Could you check a few things on this model? Use its own coordinates, in mm. A direction names the side the tool comes from. Round coordinates to 2 decimals unless told otherwise and drop trailing zeros. Loops run counter-clockwise (first coordinate to the right, second up) from the corner with the lowest first, then second, coordinate; pieces in that order, holes last. Notation, with made-up numbers: (50.25, 24) -> (106.25, 24) arc R29 cw to (106.25, 50) -> close; hole circle Ø1 at (69, 49). An arc over 180 degrees is marked (long way). Write each question's results on one line, items separated by ' | '. Start each with the question number.
1) Imagine slicing it at A-A, the plane z = -88. List the corners of the cut face in (x, y) for me, plus the area to 3 significant figures.
2) Imagine slicing it at C-C, the plane x = -29.45. List the corners of the cut face in (y, z) for me, plus the area to 3 significant figures.
3) Imagine slicing it at D-D, the plane y = 22.5. List the corners of the cut face in (x, z) for me, plus the area to 3 significant figures.
4) If I drill on probe 1 along X at (y, z) = (1, -4); probe 2 along Z at (x, y) = (-106, 1.75); probe 3 along Z at (x, y) = (-106, 0.45), over which ranges is the centre line in solid material (lowest first)?
5) Imagine slicing it at B-B, the plane y = 5. List the corners of the cut face in (x, z) for me, plus the area to 3 significant figures.
6) Which directions (+Z, -Z, +X, -X, +Y, -Y) give clear straight access to the entire face, cutting with the end or side of a thin tool? Please do faces 1 (the flat face through (-33.9, 5, -79)), 2 (the flat face through (-25, 5, -79)), 3 (the flat face through (-29, 5, -75.5)).
7) We'd pull the mould along Z, two halves only. Please class faces 4 (the flat face through (-30, 5, -82.5)), 5 (the cylindrical face through (-28.164, 4.451, -78.331)), 6 (the cylindrical face through (-0.9, 1.01, -0.86)), 7 (the flat face through (-30, 8, -77)): pulls with the +Z half, pulls with the -Z half, needs draft (parallel to the pull), parting line crosses it, or undercut.
8) For P1, Ø6, axis at x = -106, z = -4, coming from the +Y side; P2, Ø3, axis at x = -49, y = 20.5, coming from the +Z side; P3, Ø1.5, axis at x = -54, y = 16.5, coming from the -Z side, each with a flat end and sliding along its axis, tell me the tip position at first contact or that it passes through.
Autodesk Inventor part; units mm, degrees
ref_plane "Płaszczyzna konstrukcyjna2" through (-100, 0, -97) normal (-1, 0, 0) x (0, 0, 1)
ref_plane "YZ Plane" through (0, 0, 0) normal (1, 0, 0) x (0, 1, 0)
ref_plane "XZ Plane" through (0, 0, 0) normal (0, 1, 0) x (-1, 0, 0)
sketch "Szkic1" plane through (0, 0, 0) normal (0, 1, 0) x (-1, 0, 0)
  line L0 (110, 0) -> (0, 0)
  line L1 (0, 0) -> (0, -100)
  line L2 (0, -100) -> (110, -100)
  line L3 (110, -100) -> (110, 0)
  dimension "d0" = 100
  dimension "d1" = 110
extrude "Gabaryt" add sketch "Szkic1" along normal blind 2
sketch "Szkic2" plane through (0, 0, 0) normal (0, 1, 0) x (1, 0, 0)
  line L0 (0, 0) -> (0, 100)
  line L1 (-110, 0) -> (0, 0)
  line L2 (-110, 100) -> (-110, 0)
  line L3 (0, 100) -> (-110, 100)
  line L4 (-110, 50) -> (0, 50)
  line L5 (-55, 100) -> (-55, 0)
  point P0 (-4, 4)
  point P1 (-106, 4)
  point P2 (-4, 96)
  point P3 (-106, 96)
  dimension "d4" = 4
  dimension "d5" = 4
hole "Otwory montażowe" at (-4, 0, -4) at (-106, 0, -4) at (-106, 0, -96) at (-4, 0, -96) direction (0, 1, 0) diameter 2.6 end through all counterbore diameter 4.5 counterbore depth 1.5
fillet "Zaokrąglenie1" radius 3 4 edges at (0, 1, 0) (-110, 1, 0) (-110, 1, -100) (0, 1, -100)
ref_plane "Płaszczyzna konstrukcyjna2" through (-100, 0, -97) normal (-1, 0, 0) x (0, 0, 1)
sketch "Szkic4" plane through (-100, 0, -97) normal (-1, 0, 0) x (0, 0, 1)
  line L0 (0, 2) -> (94, 2)
  line L1 (0, 28.3) -> (2, 28.3)
  line L2 (2, 28.3) -> (2, 2)
  line L3 (2, 2) -> (0, 2)
  line L4 (0, 2) -> (0, 28.3)
  line L5 (19.5, 28.3) -> (21.5, 28.3)
  line L6 (21.5, 28.3) -> (21.5, 2)
  line L7 (21.5, 2) -> (19.5, 2)
  line L8 (19.5, 2) -> (19.5, 28.3)
  line L9 (0, 30.3) -> (21.5, 30.3)
  line L10 (21.5, 30.3) -> (21.5, 28.3)
  line L11 (21.5, 28.3) -> (0, 28.3)
  line L12 (0, 28.3) -> (0, 30.3)
  line L13 (-3, 2) -> (-3, 0)
  point P0 (97, 0)
  point P1 (2, 2)
  point P2 (2, 28.3)
  point P3 (19.5, 2)
  point P4 (21.5, 2)
  dimension "d20" = 2
  dimension "d21" = 2
  dimension "d22" = 2
  dimension "d23" = 17.5
  dimension "d24" = 26.3
  dimension "d25" = 3
extrude "Wyciągnięcie proste3" add sketch "Szkic4" against normal blind 55 contours L4 L1 L2 L0 | L12 L9 L10 L5 L11 L1 | L8 L5 L6 L0
sketch "Szkic5" plane through (0, 2, 0) normal (0, 1, 0) x (1, 0, 0)
  line L0 (-33.9, 82.5) -> (-25, 82.5)
  line L1 (-25, 82.5) -> (-25, 75.5)
  line L2 (-25, 75.5) -> (-33.9, 75.5)
  line L3 (-33.9, 75.5) -> (-33.9, 82.5)
  line L4 (-100, 75.5) -> (-45, 75.5)
  line L5 (-110, 97) -> (-110, 3)
  line L6 (0, 3) -> (0, 97)
  point P0 (0, 0)
  point P1 (-29.45, 82.5)
  dimension "d28" = 7
  dimension "d29" = 8.9
  dimension "d34" = 25
extrude "Wyciągnięcie proste4" add sketch "Szkic5" along normal blind 6
sketch "Szkic6" plane through (0, 8, 0) normal (0, 1, 0) x (1, 0, 0)
  line L0 (-25, 82.5) -> (-33.9, 82.5)
  line L1 (-33.9, 82.5) -> (-33.9, 75.5)
  line L2 (-33.9, 75.5) -> (-25, 75.5)
  line L3 (-25, 75.5) -> (-25, 82.5)
  line L4 (-33.9, 75.5) -> (-33.9, 82.5)
  line L5 (-33.9, 79) -> (-25, 79)
  line L6 (-29.45, 82.5) -> (-29.45, 75.5)
  point P0 (0, 0)
  point P1 (-29.45, 79)
hole "Otwór2" at (-29.45, 8, -79) direction (0, -1, 0) diameter 2.9 depth 7
equation "\"d0\" = podstawa_a"
equation "\"d1\" = podstawa_b"
equation "\"d2\" = podstawa_wys"
equation "\"d6\" = gniazdo_M2_D2"
equation "\"d8\" = gniazdo_M2_D1"
equation "\"d9\" = gniazdo_M2_glebokosc"
equation "\"d13\" = podstawa_zaokraglenie"
equation "\"d20\" = obudowa_uchwyt_grubosc"
equation "\"d21\" = d20"
equation "\"d22\" = d20"
equation "\"d23\" = obudowa_uchwyt_szerokosc_wew"
equation "\"d24\" = obudowa_uchwyt_wysokosc_wew"
equation "\"d25\" = obudowa_uchwyt_poz_z"
equation "\"d26\" = obudowa_uchwyt_kolnierz_wys"
equation "\"d28\" = podstawa_mocowanie_DC_a"
equation "\"d29\" = podstawa_mocowanie_DC_b"
equation "\"d34\" = obudowa_gniazdo_poz"
equation "\"d32\" = podstawa_mocowanie_DC_wys"
equation "\"d35\" = insert_D"
equation "\"d37\" = gniazdo_M2_D1"
equation "\"d38\" = gniazdo_M2_glebokosc"
equation "\"d40\" = insert_glebokosc"
equation "\"podstawa_a\" = 100"
equation "\"podstawa_b\" = 110"
equation "\"podstawa_wys\" = 2"
equation "\"podstawa_otwory_montazowe_poz_y\" = 4"
equation "\"podstawa_otwory_montazowe_poz_x\" = 4"
equation "\"gniazdo_M2_D1\" = 4.5"
equation "\"gniazdo_M2_glebokosc\" = 1.5"
equation "\"gniazdo_M2_D2\" = 2.6"
equation "\"obudowa_wys\" = 45"
equation "\"obudowa_grubosc\" = 2"
equation "\"obudowa_prowadnica_odsuniecie\" = 2"
equation "\"obudowa_prowadnica_grubosc\" = 2"
equation "\"obudowa_kontrolki_a\" = 38"
equation "\"obudowa_prowadnica_wys\" = 19"
equation "\"obudowa_otwory_montazowe_poz_y\" = 4"
equation "\"obudowa_otwory_montazowe_poz_x\" = 4"
equation "\"obudowa_otwory_montazowe_material_y\" = 8"
equation "\"obudowa_otwory_montazowe_material_x\" = 8"
equation "\"insert_D\" = 2.9"
equation "\"insert_glebokosc\" = 7"
equation "\"obudowa_zaokraglenie\" = 3"
equation "\"podstawa_zaokraglenie\" = 3"
equation "\"obudowa_otwory_io_wys\" = 15"
equation "\"obudowa_otwory_io_D\" = 15"
equation "\"obudowa_otwory_io1_poz\" = 55"
equation "\"obudowa_otwory_io1_wys\" = 25"
equation "\"obudowa_otwory_io1_D\" = 12"
equation "\"obudowa_otwory_io2_poz\" = 38"
equation "\"obudowa_otwory_io2_wys\" = 25"
equation "\"obudowa_otwory_io2_D\" = 12"
equation "\"obudowa_otwory_pot_D\" = 7.2"
equation "\"input_b\" = 14.4"
equation "\"input_wys\" = 10.9"
equation "\"input_a\" = 8.9"
equation "\"obudowa_MTS_otwor_D\" = 6.2"
equation "\"obudowa_pot_poz_y\" = 15"
equation "\"obudowa_s_poz_x\" = 78"
equation "\"obudowa_s_D\" = 6.2"
equation "\"obudowa_s_poz_y\" = 15"
equation "\"obudowa_s_rozstaw_y\" = 16"
equation "\"pcb_rozstaw_x\" = 92"
equation "\"pcb_rozstaw_y\" = 58"
equation "\"obudowa_pcb_grubosc_scianki\" = 6"
equation "\"pcb_grubosc_scianki\" = 6"
equation "\"pcb_poz_y\" = 29"
equation "\"pcb_wys_bloku\" = 35"
equation "\"obudowa_footswitch_poz_y\" = 68"
equation "\"obudowa_footswitch_poz_x\" = 35"
equation "\"obudowa_footswitch_D\" = 12.3"
equation "\"obudowa_led_indicator_D\" = 3.5"
equation "\"obudowa_led_indicator_poz_x\" = 55"
equation "\"obudowa_podkladka_otwory\" = 4"
equation "\"podstawa_uchwyt_grubosc\" = 3"
equation "\"podstawa_uchwyt_wysokosc\" = 15"
equation "\"obudowa_uchwyt_grubosc\" = 2"
equation "\"pbudowa_uchwyt_podciecie_wys\" = 1.5"
equation "\"obudowa_uchwyt_wysokosc_wew\" = 26.3"
equation "\"obudowa_uchwyt_szerokosc_wew\" = 17.5"
equation "\"obudowa_gniazdo_poz\" = 25"
equation "\"obudowa_uchwyt_kolnierz_wys\" = 55"
equation "\"obudowa_uchwyt_poz_y\" = 2"
equation "\"obudowa_uchwyt_poz_z\" = 3"
equation "\"obudowa_podciecie_inout_wys\" = 6"
equation "\"obudowa_podciecie_logo_wys\" = 34"
equation "\"obudowa_podciecie_logo_szerokosc\" = 25"
equation "\"obudowa_pot_pozycjonowanie_wys\" = 13"
equation "\"obudowa_pot_pozycjonowanie_szerokosc\" = 2.8"
equation "\"obudowa_pot_pozycjonowanie_glebokosc\" = 1.4"
equation "\"obudowa_led_mocowanie_wys\" = 6"
equation "\"obudowa_led_mocowanie_poz\" = 46"
equation "\"obudowa_led_mocowanie_D\" = 5.5"
equation "\"obudowa_led_mocowanie_grubosc\" = 8"
equation "\"holder_led_grubosc\" = 2.5"
equation "\"holder_led_dlugosc\" = 28"
equation "\"holder_led_uchwyt_D\" = 5"
equation "\"holder_led_uchwyt_wysokosc\" = 5"
equation "\"holder_led_uchwyt_szerokosc\" = 8"
equation "\"holder_gniazdo_b\" = 5"
equation "\"holder_gniazdo_grubosc\" = 2.5"
equation "\"holder_gniazdo_a\" = 28"
equation "\"podstawa_mocowanie_DC_a\" = 7"
equation "\"podstawa_mocowanie_DC_b\" = 8.9"
equation "\"podstawa_mocowanie_DC_wys\" = 6"
equation "\"holder_gniazdo_odleglosc_miedzy_ramionami\" = 9.2"
equation "\"holder_gniazdo_grubosc_ramion\" = 1.5"
equation "\"holder_gniazdo_wys\" = 8"
equation "\"holder_gniazdo_uchwyt_poz\" = 5"
properties part number "podstawa"
Checked values:
1) outline: (-110, 0) -> (0, 0) -> (0, 2) -> (-110, 2) -> close; (-100, 28.3) -> (-45, 28.3) -> (-45, 30.3) -> (-100, 30.3) -> close | area: 330 mm^2
2) outline: (0, -100) -> (2, -100) -> (2, -82.5) -> (8, -82.5) -> (8, -80.45) -> (1, -80.45) -> (1, -77.55) -> (8, -77.55) -> (8, -75.5) -> (2, -75.5) -> (2, 0) -> (0, 0) -> close | area: 222 mm^2
3) outline: (-100, -97) -> (-45, -97) -> (-45, -95) -> (-100, -95) -> close; (-100, -77.5) -> (-45, -77.5) -> (-45, -75.5) -> (-100, -75.5) -> close | area: 220 mm^2
4) probe 1: -110 to -108.25, -103.75 to -6.25, -1.75 to 0 | probe 2: -100 to -97.3, -94.7 to -5.3, -2.7 to 0 | probe 3: -100 to -98.25, -93.75 to -6.25, -1.75 to 0
5) outline: (-100, -97) -> (-45, -97) -> (-45, -95) -> (-100, -95) -> close; (-100, -77.5) -> (-45, -77.5) -> (-45, -75.5) -> (-100, -75.5) -> close; (-33.9, -82.5) -> (-25, -82.5) -> (-25, -75.5) -> (-33.9, -75.5) -> close; hole circle Ø2.9 at (-29.45, -79) | area: 276 mm^2
6) face 1: +Z, -Z, +Y | face 2: +Z, -Z, +X, +Y | face 3: +Z, +X, -X, +Y
7) face 4: pulls with the -Z half | face 5: undercut | face 6: pulls with the +Z half | face 7: needs draft
8) P1: y = 2 | P2: z = -75.5 | P3: z = -97
